Source: CAD feature listing. Evaluate the final solid. Frame: model axes, mm. Face numbers are marked on the shaded views. A direction names the side the tool comes from. Give positions to 0.01 mm unless a question says otherwise; leave off trailing zeros. Loops run counter-clockwise (first coordinate to the right, second up) from the corner with the lowest first, then second, coordinate; pieces in that order, holes last. Notation, with made-up numbers: (3, 55.25) -> (48, 55.25) arc R35 cw to (48, 91.25) -> close; hole circle Ø10 at (38, 48.25). An arc over 180 degrees is marked (long way). Return JSON: item names as keys, results as strings. Group by question number.
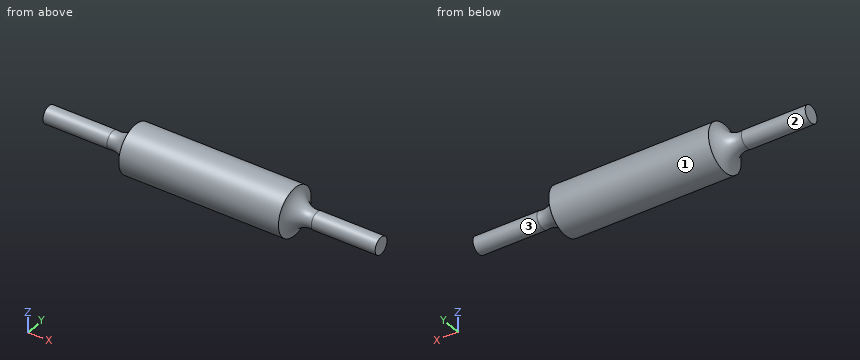
```python
from build123d import *


with BuildPart() as part:
    # Esboço1 → Revolução1 (revolve)
    with BuildSketch(Plane(origin=(0, 0, 0), x_dir=(1, 0, 0), z_dir=(0, 1, 0))):
        with BuildLine():
            Line((-25, -7.5), (25, -7.5))
            ThreePointArc((25, -7.5), (27.50675077, -3.65233677), (32, -2.704168477))
            Line((32, -2.704168477), (52, -2.704168477))
            Line((52, -2.704168477), (52, 0))
            Line((52, 0), (-52, 0))
            Line((-52, 0), (-52, -2.704168477))
            Line((-52, -2.704168477), (-32, -2.704168477))
            ThreePointArc((-32, -2.704168477), (-27.50675077, -3.65233677), (-25, -7.5))
        make_face()
    revolve(axis=Axis((-4.5, 0, 0), (1, 0, 0)))


solid = part.part
```
1) Cut plane D-D on x = -3. Return loops of the section in (y, z).
2) Material intervals for line 1 (Y direction, x = -5.5, z = -0.5); line 2 (X direction, y = 7, z = 1.5); line 3 (Y direction, x = -31, z = 0.5), sorted ascending.
3) Reachability of the marked faces 1, 2 and 3 from +Z, -Z, +X, -X, +Y, -Y: full face, straight path, thin tool, end or side. Return the list, or none.
4) Cut plane A-A on z = 0. Return loops of the section in (x, y), then the cut area to 3 significant figures.
5) Cut plane C-C on x = -38. Return loops of the section in (y, z), then the cut area to 3 significant figures.
6) Contact query for flat-ended pins moving along their axis: P1, Ø3, axis at x = 17, z = -4, coming from the +Y side; P2, Ø2, axis at y = 4, z = 1, coming from the +X side; P3, Ø2, axis at x = -37, y = 0.5, coming from the +Z side. Output: stop coordinate, or through.
Calculated:
{
 "1": {"outline": "circle Ø15 at (0, 0)"},
 "2": {"line 1": "-7.48 to 7.48", "line 2": "-25.07 to 25.07", "line 3": "-2.55 to 2.55"},
 "3": {"face 1": "+X, -X", "face 2": "-X", "face 3": "+X"},
 "4": {"outline": "(-52, -2.7) -> (-32, -2.7) arc R6 cw to (-25, -7.5) -> (25, -7.5) arc R6 cw to (32, -2.7) -> (52, -2.7) -> (52, 2.7) -> (32, 2.7) arc R6 cw to (25, 7.5) -> (-25, 7.5) arc R6 cw to (-32, 2.7) -> (-52, 2.7) -> close", "area": "1,070 mm2"},
 "5": {"outline": "circle Ø5.41 at (0, 0)", "area": "23.0 mm2"},
 "6": {"P1": "y = 7.07", "P2": "x = 28.45", "P3": "z = 2.7"}
}
